Can you work these out from the model? Positions are in its coordinate system, mm. Round coordinates to 2 decimals unless told otherwise and drop trailing zeros. Loops run counter-clockwise (first coordinate to the right, second up) from the corner with the lowest first, then second, coordinate; pieces in that order, holes last. Notation, with made-up numbers: (70, 77) -> (94, 77) arc R25 cw to (94, 113) -> close; hole circle Ø8 at (62, 64). An arc over 180 degrees is marked (long way). Write each question's results on one line, items separated by ' | '.
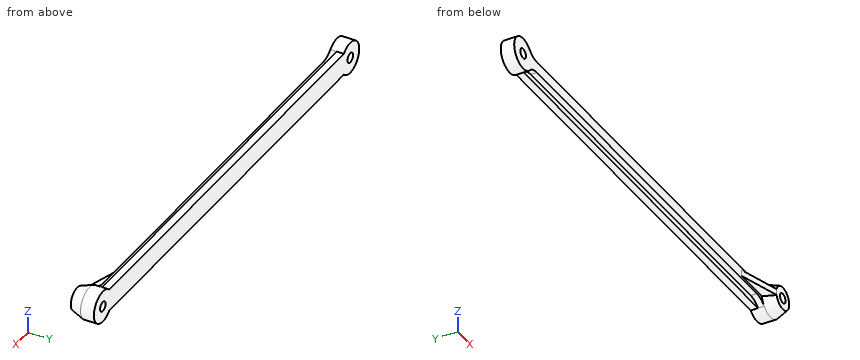
from build123d import *
from build123d.topology import SkipClean

# Parameters (mm, degrees)
SKETCH1_R           = 2
BOSS_EXTRUDE1_DEPTH = 5.5
CUT_EXTRUDE1_DEPTH  = 2.5
SKETCH4_R           = 6.5
SKETCH3_R           = 4.68
SKETCH5_R           = 2
CUT_EXTRUDE2_DEPTH  = 187.908400029
BOSS_EXTRUDE2_DEPTH = 1.25


with BuildPart() as part:
    # Sketch1 → Boss-Extrude1 (new body)
    with BuildSketch(Plane(origin=(0, 0, 0), x_dir=(1, 0, 0), z_dir=(0, 1, 0))):
        with BuildLine():
            Line((-175.30958424, 4.5), (-4.69041576, 4.5))
            ThreePointArc((-4.69041576, 4.5), (6.5, 0), (-4.69041576, -4.5))
            Line((-4.69041576, -4.5), (-175.30958424, -4.5))
            ThreePointArc((-175.30958424, -4.5), (-186.5, 0), (-175.30958424, 4.5))
        make_face()
        with Locations(Location((0, 0, 0), (0, 0, 270))):
            Circle(SKETCH1_R, mode=Mode.SUBTRACT)
        with Locations(Location((-180, 0, 0), (0, 0, 270))):
            Circle(SKETCH1_R, mode=Mode.SUBTRACT)
    extrude(amount=BOSS_EXTRUDE1_DEPTH)

    # Sketch2 → Cut-Extrude1 (cut)
    with BuildSketch(Plane.XZ):
        with BuildLine():
            Line((-9.96713349, 2.25), (-170.03286651, 2.25))
            ThreePointArc((-170.03286651, 2.25), (-172.901064987, 2.835978332), (-175.30958424, 4.5))
            Line((-175.30958424, 4.5), (-4.69041576, 4.5))
            ThreePointArc((-4.69041576, 4.5), (-7.098935013, 2.835978332), (-9.96713349, 2.25))
        make_face()
        with BuildLine():
            Line((-9.96713349, -2.25), (-170.03286651, -2.25))
            ThreePointArc((-170.03286651, -2.25), (-172.901064987, -2.835978332), (-175.30958424, -4.5))
            Line((-175.30958424, -4.5), (-4.69041576, -4.5))
            ThreePointArc((-4.69041576, -4.5), (-7.098935013, -2.835978332), (-9.96713349, -2.25))
        make_face()
    extrude(amount=-CUT_EXTRUDE1_DEPTH, mode=Mode.SUBTRACT)

    # Sketch4 → Loft1 section 0
    with BuildSketch(Plane.XZ):
        Circle(SKETCH4_R)
    # Sketch3 → Loft1 section 1
    with BuildSketch(Plane(origin=(0, -5, 0), x_dir=(-1, 0, 0), z_dir=(0, -1, 0))):
        Circle(SKETCH3_R)
    loft()

    # Sketch5 → Cut-Extrude2 (cut, through all)
    with SkipClean():  # the faces are left unmerged after this step: merging them gives an invalid solid
        with BuildSketch(Plane.XZ.offset(5)):
            with Locations(Location((0, 0, 0), (0, 0, 270))):
                Circle(SKETCH5_R)
        extrude(amount=-CUT_EXTRUDE2_DEPTH, mode=Mode.SUBTRACT)

    # Sketch6 → Boss-Extrude2 (add, symmetric)
    with SkipClean():  # the faces are left unmerged after this step: merging them gives an invalid solid
        with BuildSketch(Plane.XY):
            Polygon((-3.080000032, 0), (-21.280000032, 0), (-4.680000032, -5), (-3.080000032, -5), align=None)
        extrude(amount=BOSS_EXTRUDE2_DEPTH, both=True)


solid = part.part
1. If we section it at D-D (x = -180): List the corners of the cut face in (y, z) for me, then the cut area to 3 significant figures.
Final values:
outline: (0, -6.5) -> (5.5, -6.5) -> (5.5, -2) -> (0, -2) -> close; (0, 2) -> (5.5, 2) -> (5.5, 6.5) -> (0, 6.5) -> close | area: 49.5 mm2
2. Please list where these lines run through material, in increasing order: line 1 (X direction, y = 3.5, z = 0); line 2 (Z direction, x = 0, y = 1.5); line 3 (Z direction, x = -173, y = 3.75). Write a range as from..to.
Final values:
line 1: -186.5..-182, -178..-2, 2..6.5 | line 2: -6.5..-2, 2..6.5 | line 3: -4.5..4.5
3. If we section it at A-A (x = 0): List the corners of the cut face in (y, z) for me.
Final values:
outline: (-5, -4.68) -> (0, -6.5) -> (5.5, -6.5) -> (5.5, -2) -> (-5, -2) -> close; (-5, 2) -> (5.5, 2) -> (5.5, 6.5) -> (0, 6.5) -> (-5, 4.68) -> close
4. If we section it at C-C (y = -2.5): List the corners of the cut face in (x, z) for me, then the cut area to 3 significant figures.
Final values:
outline: (-12.98, -1.25) -> (-5.45, -1.25) arc R5.59 ccw (long way) to (-5.45, 1.25) -> (-12.98, 1.25) -> close; hole circle Ø4 at (0, 0) | area: 104 mm2
5. Will these pins go through, and if not, where does the flat tip stop? pin 1 (1.2 mm diameter, centred on x = -125.5, y = 1.5, fed in from +Z); pin 2 (4 mm diameter, centred on x = -124.5, z = -2, fed in from -Y); pin 3 (4 mm diameter, centred on y = 4, z = -0.5, fed in from +X); pin 4 (3.5 mm diameter, centred on x = 0, z = 0, fed in from -Y).
Final values:
pin 1: z = 2.25 | pin 2: y = 0 | pin 3: x = 6.5 | pin 4: through
6. If we section it at B-B (x = -78): List the corners of the cut face in (y, z) for me.
Final values:
outline: (0, -2.25) -> (2.5, -2.25) -> (2.5, -4.5) -> (5.5, -4.5) -> (5.5, 4.5) -> (2.5, 4.5) -> (2.5, 2.25) -> (0, 2.25) -> close
